```python
from build123d import *

# Parameters (mm, degrees)
SKETCH1_W           = 42.9
SKETCH1_H           = 40.5
SKETCH1_R           = 1.55
BOSS_EXTRUDE1_DEPTH = 1.6
FILLET1_R           = 2
SKETCH2_W           = 5.4
SKETCH2_H           = 4.1
BOSS_EXTRUDE2_DEPTH = 2.5
SKETCH3_W           = 20.5
SKETCH3_H           = 2.56
BOSS_EXTRUDE3_DEPTH = 2.3


with BuildPart() as part:
    # Sketch1 → Boss-Extrude1 (new body)
    with BuildSketch(Plane(origin=(0, 0, 0), x_dir=(1, 0, 0), z_dir=(0, 1, 0))):
        with Locations((-8.819274306, 9.105101592)):
            Rectangle(SKETCH1_W, SKETCH1_H)
        with Locations((-22.969274306, 22.055101592)):
            Circle(SKETCH1_R, mode=Mode.SUBTRACT)
        with Locations((5.330725694, -3.844898408)):
            Circle(SKETCH1_R, mode=Mode.SUBTRACT)
    extrude(amount=BOSS_EXTRUDE1_DEPTH)

    # Fillet1
    fillet1_edges = [part.edges().sort_by_distance(p)[0] for p in [
        (-30.269274306, 0.8, -29.355101592),
        (12.630725694, 0.8, -29.355101592),
        (12.630725694, 0.8, 11.144898408),
        (-30.269274306, 0.8, 11.144898408),
    ]]
    fillet(fillet1_edges, radius=FILLET1_R)

    # Sketch2 → Boss-Extrude2 (add)
    with BuildSketch(Plane(origin=(0, 1.6, 0), x_dir=(1, 0, 0), z_dir=(0, 1, 0))):
        with Locations((1.130725694, 18.505101592)):
            Rectangle(SKETCH2_W, SKETCH2_H)
    extrude(amount=BOSS_EXTRUDE2_DEPTH)

    # Sketch3 → Boss-Extrude3 (add)
    with BuildSketch(Plane.XZ):
        with Locations((-11.419274306, 4.614898408)):
            Rectangle(SKETCH3_W, SKETCH3_H)
    extrude(amount=BOSS_EXTRUDE3_DEPTH)


solid = part.part
```
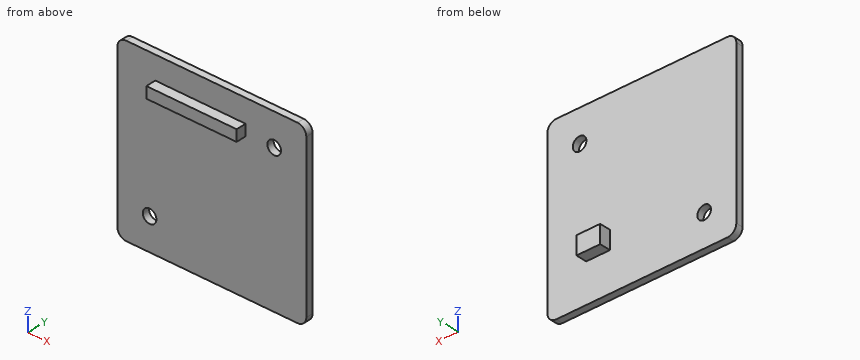
Could you check a few things on this model? Use its own coordinates, in mm. Give positions to 0.01 mm unless a question says otherwise; leave off trailing zeros. Loops run counter-clockwise (first coordinate to the right, second up) from the corner with the lowest first, then second, coordinate; pieces in that order, holes last. Notation, with made-up numbers: (71, -12.75) - (110, -12.75) arc R10 cw to (110, 2.25) - close; hole circle Ø7 at (-34.5, 17.25). An arc over 180 degrees is marked (long way). Answer in a Markdown table with one row per item. Add a question column.
Q1. Please list where these lines run through material, in increasing order: L1, parallel to Z at x = -5, y = -0.75; L2, parallel to Z at x = -22.5, y = 0.5; L3, parallel to Y at x = -28, z = 0. Write a range as from..to.
Q2. If we section it at C-C (x = -23.5): List the corners of the cut face in (y, z) for me.
Q3. If we section it at D-D (y = 3.5): List the corners of the cut face in (x, z) for me, plus the area to 3 significant figures.
Q4. For pin 1 (0.7 mm diameter, centred on y = -1.5, z = 5, fed in from +X); pin 2 (1.5 mm diameter, centred on x = -22.5, z = -3.5, fed in from +Y); pin 3 (4 mm diameter, centred on x = 2.5, z = -23, fed in from -Y), each with a flat end and sliding along its axis, tell me the tip position at first contact or that it passes through.
Q5. If we section it at A-A (x = -18.5): List the corners of the cut face in (y, z) for me.
Q6. If we section it at B-B (z = -20): List the corners of the cut face in (x, y) for me.
The answers:
| question | item | result |
|---|---|---|
| 1 | L1 | z = 3.33..5.89 |
| 1 | L2 | z = -29.36..-23.53, -20.58..11.14 |
| 1 | L3 | y = 0..1.6 |
| 2 | outline | (0, -29.36) - (1.6, -29.36) - (1.6, -23.51) - (0, -23.51) - close; (0, -20.6) - (1.6, -20.6) - (1.6, 11.14) - (0, 11.14) - close |
| 3 | outline | (-1.57, -20.56) - (3.83, -20.56) - (3.83, -16.46) - (-1.57, -16.46) - close |
| 3 | area | 22.1 mm^2 |
| 4 | pin 1 | stops at x = -1.17 |
| 4 | pin 2 | stops at y = 1.6 |
| 4 | pin 3 | stops at y = 0 |
| 5 | outline | (-2.3, 3.33) - (0, 3.33) - (0, -29.36) - (1.6, -29.36) - (1.6, 11.14) - (0, 11.14) - (0, 5.89) - (-2.3, 5.89) - close |
| 6 | outline | (-30.27, 0) - (12.63, 0) - (12.63, 1.6) - (3.83, 1.6) - (3.83, 4.1) - (-1.57, 4.1) - (-1.57, 1.6) - (-30.27, 1.6) - close |
